Check sheet for the modelled part. Datum: model origin and axes. Units: mm. Face numbers are marked on the shaded views. A direction names the side the tool comes from. Round coordinates to 2 decimals unless told otherwise and drop trailing zeros. Loops run counter-clockwise (first coordinate to the right, second up) from the corner with the lowest first, then second, coordinate; pieces in that order, holes last. Notation, with made-up numbers: (82.5, -38) - (105.5, -38) arc R30 ccw to (105.5, -12) - close; hole circle Ø10 at (80.25, 86). An arc over 180 degrees is marked (long way). Answer in a Markdown table with one row per item. Add a question column.
(1) Access from +Z, -Z, +X, -X, +Y, -Y to the whole of each face (thin tool, end or side, straight path). Record for the marked faces 4 and 5.
(2) Cross-section at A-A on y = 4.75. Enter the section's corners in (x, z).
(3) Mould release check, pull along Z, two halves, no side actions. Record for the marked faces 1, 2 and 3: +Z half, -Z half, draft (parallel to the pull), parting line (faces both ways), or undercut.
(4) Thickness scan on line 1 along Z through (x, y) = (27, 14.75); line 2 along Z through (x, y) = (3, 9.25); line 3 along X through (y, z) = (12.5, 19). Record the ranges inside material, lowest first.
(5) Gauge pin test, flat ends, axial feed: pin 1 (0.6 mm diameter, centred on x = -31, y = 18, fed in from +Z); pin 2 (0.9 mm diameter, centred on x = -32.5, y = 3, fed in from -Z); pin 3 (3 mm diameter, centred on x = -21, z = -6.5, fed in from +Y). Record the tip position at first contact, or that the pin passes through.
(6) Cross-section at B-B on y = 16.25. Enter the section's corners in (x, z).
from build123d import *

# Parameters (mm, degrees)
SKETCH1_W           = 61
SKETCH1_H           = 41
BOSS_EXTRUDE1_DEPTH = 23
SHELL1_T            = 3
SKETCH2_W           = 11
SKETCH2_H           = 6.5
CUT_EXTRUDE1_DEPTH  = 72.953109731
SKETCH3_W           = 61
SKETCH3_H           = 1.8
BOSS_EXTRUDE2_DEPTH = 10
SKETCH4_R           = 1.05
CUT_EXTRUDE2_DEPTH  = 41
SKETCH5_R           = 1.05
CUT_EXTRUDE3_DEPTH  = 61
FILLET1_SIZE        = 1
FILLET1_SIZE_2      = 3
FILLET2_R           = 3


with BuildPart() as part:
    # Sketch1 → Boss-Extrude1 (new body)
    with BuildSketch(Plane(origin=(0, 0, 0), x_dir=(1, 0, 0), z_dir=(0, 1, 0))):
        Rectangle(SKETCH1_W, SKETCH1_H)
    extrude(amount=BOSS_EXTRUDE1_DEPTH)

    # Shell1
    shell1_openings = [part.faces().sort_by_distance(p)[0] for p in [
        (0, 23, 0),
    ]]
    offset(amount=SHELL1_T, openings=shell1_openings, kind=Kind.INTERSECTION)

    # Sketch2 → Cut-Extrude1 (cut, through all)
    with BuildSketch(Plane(origin=(-30.5, 0, 0), x_dir=(0, 0, -1), z_dir=(1, 0, 0))):
        with Locations((-6.5, 4.5)):
            Rectangle(SKETCH2_W, SKETCH2_H)
    extrude(amount=-CUT_EXTRUDE1_DEPTH, mode=Mode.SUBTRACT)

    # Sketch3 → Boss-Extrude2 (add)
    with BuildSketch(Plane(origin=(0, 0, 0), x_dir=(1, 0, 0), z_dir=(0, 1, 0))):
        with Locations((0, 19.6)):
            Rectangle(SKETCH3_W, SKETCH3_H)
        with Locations((0, -19.6)):
            Rectangle(SKETCH3_W, SKETCH3_H)
    extrude(amount=BOSS_EXTRUDE2_DEPTH)

    # Sketch4 → Cut-Extrude2 (cut)
    with BuildSketch(Plane.XY.offset(-20.5)):
        with Locations((-30, 18.1)):
            Circle(SKETCH4_R)
        with Locations((30, 18.1)):
            Circle(SKETCH4_R)
    extrude(amount=CUT_EXTRUDE2_DEPTH, mode=Mode.SUBTRACT)

    # Sketch5 → Cut-Extrude3 (cut)
    with BuildSketch(Plane(origin=(-30.5, 0, 0), x_dir=(0, 0, -1), z_dir=(1, 0, 0))):
        with Locations((-20, 18.1)):
            Circle(SKETCH5_R)
        with Locations((20, 18.1)):
            Circle(SKETCH5_R)
    extrude(amount=CUT_EXTRUDE3_DEPTH, mode=Mode.SUBTRACT)

    # Fillet1
    # an asymmetric fillet: 3, 1 mm, written as the material it takes off along each edge
    with BuildSketch(Plane(origin=(30.5, 23, 20.5), x_dir=(0, 0, 1), z_dir=(-1, 0, 0)), Plane(origin=(-30.5, 23, -20.5), x_dir=(0, 0, -1), z_dir=(1, 0, 0))) as fillet1_piece_1:
        with BuildLine():
            Bezier((FILLET1_SIZE, 0), (0, 0), (0, -FILLET1_SIZE_2), weights=[1, 0.707106781, 1])
            Line((0, -FILLET1_SIZE_2), (-0.06, -3))
            Line((-0.06, -3), (-0.06, 0.06))
            Line((-0.06, 0.06), (1, 0.06))
            Line((1, 0.06), (FILLET1_SIZE, 0))
        make_face()
    extrude(amount=61, mode=Mode.SUBTRACT)
    with BuildSketch(Plane(origin=(30.5, 23, -20.5), x_dir=(1, 0, 0), z_dir=(0, 0, 1)), Plane(origin=(-30.5, 23, 20.5), x_dir=(-1, 0, 0), z_dir=(0, 0, -1))) as fillet1_piece_2:
        with BuildLine():
            Bezier((FILLET1_SIZE, 0), (0, 0), (0, -FILLET1_SIZE_2), weights=[1, 0.707106781, 1])
            Line((0, -FILLET1_SIZE_2), (-0.06, -3))
            Line((-0.06, -3), (-0.06, 0.06))
            Line((-0.06, 0.06), (1, 0.06))
            Line((1, 0.06), (FILLET1_SIZE, 0))
        make_face()
    extrude(amount=41, mode=Mode.SUBTRACT)
    with BuildSketch(Plane(origin=(38, 23, 20.5), x_dir=(0, 0, 1), z_dir=(-1, 0, 0))) as fillet1_piece_3a_section:
        with BuildLine():
            Bezier((FILLET1_SIZE, 0), (0, 0), (0, -FILLET1_SIZE_2), weights=[1, 0.707106781, 1])
            Line((0, -FILLET1_SIZE_2), (-0.06, -3))
            Line((-0.06, -3), (-0.06, 0.06))
            Line((-0.06, 0.06), (1, 0.06))
            Line((1, 0.06), (FILLET1_SIZE, 0))
        make_face()
    fillet1_piece_3a = extrude(amount=68.5, mode=Mode.PRIVATE)
    fillet1_piece_3a = split(fillet1_piece_3a, bisect_by=Plane(origin=(30.5, 22.211737764, 20.689651293), z_dir=(1, 0, 0)), keep=Keep.TOP, mode=Mode.PRIVATE)
    with BuildSketch(Plane(origin=(30.5, 23, -20.5), x_dir=(1, 0, 0), z_dir=(0, 0, 1))) as fillet1_piece_3b_section:
        with BuildLine():
            Bezier((FILLET1_SIZE, 0), (0, 0), (0, -FILLET1_SIZE_2), weights=[1, 0.707106781, 1])
            Line((0, -FILLET1_SIZE_2), (-0.06, -3))
            Line((-0.06, -3), (-0.06, 0.06))
            Line((-0.06, 0.06), (1, 0.06))
            Line((1, 0.06), (FILLET1_SIZE, 0))
        make_face()
    fillet1_piece_3b = extrude(amount=48.5, mode=Mode.PRIVATE)
    fillet1_piece_3b = split(fillet1_piece_3b, bisect_by=Plane(origin=(30.689651156, 22.211737177, 20.5), z_dir=(0, 0, 1)), keep=Keep.TOP, mode=Mode.PRIVATE)
    fillet1_piece_3 = fillet1_piece_3a & fillet1_piece_3b
    add(fillet1_piece_3, mode=Mode.SUBTRACT)
    with BuildSketch(Plane(origin=(-30.5, 23, 28), x_dir=(-1, 0, 0), z_dir=(0, 0, -1))) as fillet1_piece_4a_section:
        with BuildLine():
            Bezier((FILLET1_SIZE, 0), (0, 0), (0, -FILLET1_SIZE_2), weights=[1, 0.707106781, 1])
            Line((0, -FILLET1_SIZE_2), (-0.06, -3))
            Line((-0.06, -3), (-0.06, 0.06))
            Line((-0.06, 0.06), (1, 0.06))
            Line((1, 0.06), (FILLET1_SIZE, 0))
        make_face()
    fillet1_piece_4a = extrude(amount=48.5, mode=Mode.PRIVATE)
    fillet1_piece_4a = split(fillet1_piece_4a, bisect_by=Plane(origin=(-30.689651293, 22.211737761, 20.5), z_dir=(0, 0, 1)), keep=Keep.TOP, mode=Mode.PRIVATE)
    with BuildSketch(Plane(origin=(30.5, 23, 20.5), x_dir=(0, 0, 1), z_dir=(-1, 0, 0))) as fillet1_piece_4b_section:
        with BuildLine():
            Bezier((FILLET1_SIZE, 0), (0, 0), (0, -FILLET1_SIZE_2), weights=[1, 0.707106781, 1])
            Line((0, -FILLET1_SIZE_2), (-0.06, -3))
            Line((-0.06, -3), (-0.06, 0.06))
            Line((-0.06, 0.06), (1, 0.06))
            Line((1, 0.06), (FILLET1_SIZE, 0))
        make_face()
    fillet1_piece_4b = extrude(amount=68.5, mode=Mode.PRIVATE)
    fillet1_piece_4b = split(fillet1_piece_4b, bisect_by=Plane(origin=(-30.5, 22.211737179, 20.689651156), z_dir=(-1, 0, 0)), keep=Keep.TOP, mode=Mode.PRIVATE)
    fillet1_piece_4 = fillet1_piece_4a & fillet1_piece_4b
    add(fillet1_piece_4, mode=Mode.SUBTRACT)
    with BuildSketch(Plane(origin=(-30.5, 23, -20.5), x_dir=(0, 0, -1), z_dir=(1, 0, 0))) as fillet1_piece_5a_section:
        with BuildLine():
            Bezier((FILLET1_SIZE, 0), (0, 0), (0, -FILLET1_SIZE_2), weights=[1, 0.707106781, 1])
            Line((0, -FILLET1_SIZE_2), (-0.06, -3))
            Line((-0.06, -3), (-0.06, 0.06))
            Line((-0.06, 0.06), (1, 0.06))
            Line((1, 0.06), (FILLET1_SIZE, 0))
        make_face()
    fillet1_piece_5a = extrude(amount=68.5, mode=Mode.PRIVATE)
    fillet1_piece_5a = split(fillet1_piece_5a, bisect_by=Plane(origin=(30.5, 22.211737179, -20.689651156), z_dir=(1, 0, 0)), keep=Keep.TOP, mode=Mode.PRIVATE)
    with BuildSketch(Plane(origin=(30.5, 23, -28), x_dir=(1, 0, 0), z_dir=(0, 0, 1))) as fillet1_piece_5b_section:
        with BuildLine():
            Bezier((FILLET1_SIZE, 0), (0, 0), (0, -FILLET1_SIZE_2), weights=[1, 0.707106781, 1])
            Line((0, -FILLET1_SIZE_2), (-0.06, -3))
            Line((-0.06, -3), (-0.06, 0.06))
            Line((-0.06, 0.06), (1, 0.06))
            Line((1, 0.06), (FILLET1_SIZE, 0))
        make_face()
    fillet1_piece_5b = extrude(amount=48.5, mode=Mode.PRIVATE)
    fillet1_piece_5b = split(fillet1_piece_5b, bisect_by=Plane(origin=(30.689651293, 22.211737761, -20.5), z_dir=(0, 0, -1)), keep=Keep.TOP, mode=Mode.PRIVATE)
    fillet1_piece_5 = fillet1_piece_5a & fillet1_piece_5b
    add(fillet1_piece_5, mode=Mode.SUBTRACT)
    with BuildSketch(Plane(origin=(-38, 23, -20.5), x_dir=(0, 0, -1), z_dir=(1, 0, 0))) as fillet1_piece_6a_section:
        with BuildLine():
            Bezier((FILLET1_SIZE, 0), (0, 0), (0, -FILLET1_SIZE_2), weights=[1, 0.707106781, 1])
            Line((0, -FILLET1_SIZE_2), (-0.06, -3))
            Line((-0.06, -3), (-0.06, 0.06))
            Line((-0.06, 0.06), (1, 0.06))
            Line((1, 0.06), (FILLET1_SIZE, 0))
        make_face()
    fillet1_piece_6a = extrude(amount=68.5, mode=Mode.PRIVATE)
    fillet1_piece_6a = split(fillet1_piece_6a, bisect_by=Plane(origin=(-30.5, 22.211737764, -20.689651293), z_dir=(-1, 0, 0)), keep=Keep.TOP, mode=Mode.PRIVATE)
    with BuildSketch(Plane(origin=(-30.5, 23, 20.5), x_dir=(-1, 0, 0), z_dir=(0, 0, -1))) as fillet1_piece_6b_section:
        with BuildLine():
            Bezier((FILLET1_SIZE, 0), (0, 0), (0, -FILLET1_SIZE_2), weights=[1, 0.707106781, 1])
            Line((0, -FILLET1_SIZE_2), (-0.06, -3))
            Line((-0.06, -3), (-0.06, 0.06))
            Line((-0.06, 0.06), (1, 0.06))
            Line((1, 0.06), (FILLET1_SIZE, 0))
        make_face()
    fillet1_piece_6b = extrude(amount=48.5, mode=Mode.PRIVATE)
    fillet1_piece_6b = split(fillet1_piece_6b, bisect_by=Plane(origin=(-30.689651156, 22.211737177, -20.5), z_dir=(0, 0, -1)), keep=Keep.TOP, mode=Mode.PRIVATE)
    fillet1_piece_6 = fillet1_piece_6a & fillet1_piece_6b
    add(fillet1_piece_6, mode=Mode.SUBTRACT)

    # Fillet2
    fillet2_edges = [part.edges().sort_by_distance(p)[0] for p in [
        (33.5, 10, 23.5),
        (-33.5, 10, 23.5),
        (-33.5, 10, -23.5),
        (33.5, 10, -23.5),
    ]]
    fillet(fillet2_edges, radius=FILLET2_R)


solid = part.part
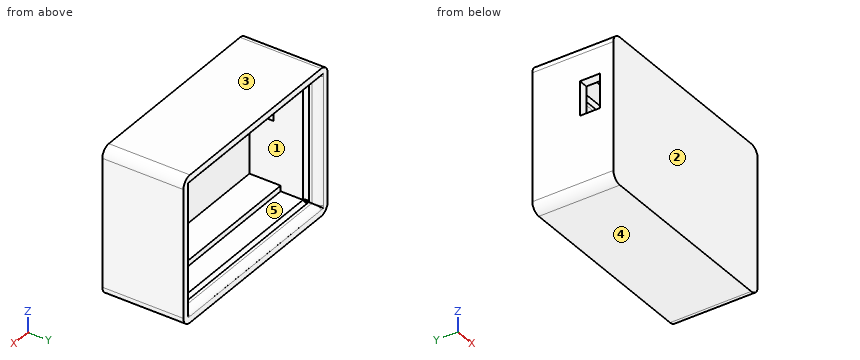
Answers:
| question | item | result |
|---|---|---|
| 1 | face 4 | -Z, +X, -X, +Y, -Y |
| 1 | face 5 | +Y |
| 2 | outline | (-33.5, -20.5) arc R3 ccw to (-30.5, -23.5) - (30.5, -23.5) arc R3 ccw to (33.5, -20.5) - (33.5, 20.5) arc R3 ccw to (30.5, 23.5) - (-30.5, 23.5) arc R3 ccw to (-33.5, 20.5) - (-33.5, 12) - (-30.5, 12) - (-30.5, 18.7) - (30.5, 18.7) - (30.5, -18.7) - (-30.5, -18.7) - (-30.5, 1) - (-33.5, 1) - close |
| 3 | face 1 | undercut |
| 3 | face 2 | draft |
| 3 | face 3 | +Z half |
| 4 | line 1 | z = -23.5 to -20.5, 20.5 to 23.5 |
| 4 | line 2 | z = -23.5 to -18.7, 18.7 to 23.5 |
| 4 | line 3 | x = -33.5 to -30.5, 30.5 to 33.5 |
| 5 | pin 1 | stops at z = 23.49 |
| 5 | pin 2 | stops at z = -23.07 |
| 5 | pin 3 | stops at y = 0 |
| 6 | outline | (-33.5, -20.5) arc R3 ccw to (-30.5, -23.5) - (30.5, -23.5) arc R3 ccw to (33.5, -20.5) - (33.5, 20.5) arc R3 ccw to (30.5, 23.5) - (-30.5, 23.5) arc R3 ccw to (-33.5, 20.5) - close; hole (-30.5, -20.5) - (30.5, -20.5) - (30.5, 20.5) - (-30.5, 20.5) - close |
